```python
from build123d import *

# Parameters (mm, degrees)
F0_W     = 19.05
F0_H     = 184.15
F1_DEPTH = 50.8
F2_W     = 12.7
F2_H     = 25.4
F3_DEPTH = 12.7
F4_W     = 12.7
F4_H     = 25.4
F5_DEPTH = 12.7
F6_R     = 6.34999


# Not quite as in the source:
# - a fillet or chamfer is up to 0.001 mm smaller than in the source, because OpenCascade refuses the exact size


with BuildPart() as f1:
    # F0 (on Top) → F1 (new body)
    with BuildSketch(Plane.XY):
        Rectangle(F0_W, F0_H)
    extrude(amount=-F1_DEPTH)

    # F2 (on face) → F3 (join)
    with BuildSketch(Plane.XZ.offset(92.075)):
        with Locations((0, -25.4)):
            Rectangle(F2_W, F2_H)
    extrude(amount=F3_DEPTH)

    # F4 (on face) → F5 (join)
    with BuildSketch(Plane(origin=(0, 92.075, 0), x_dir=(-1, 0, 0), z_dir=(0, 1, 0))):
        with Locations((0, -25.4)):
            Rectangle(F4_W, F4_H)
    extrude(amount=F5_DEPTH)

    # F6 (radius 6.35 in the source; OpenCascade refuses exactly that, so slightly less here)
    f6_edges = [f1.edges().sort_by_distance(p)[0] for p in [
        (6.35, 98.425, -12.7),
        (-6.35, 98.425, -12.7),
        (-6.35, 98.425, -38.1),
        (6.35, 98.425, -38.1),
        (-6.35, -98.425, -12.7),
        (6.35, -98.425, -12.7),
        (-6.35, -98.425, -38.1),
        (6.35, -98.425, -38.1),
    ]]
    fillet(f6_edges, radius=F6_R)


solid = f1.part
```
Can you work these out from the model? Positions are in its coordinate system, mm. A direction names the side the tool comes from. Round coordinates to 2 decimals unless told otherwise and drop trailing zeros. Loops run counter-clockwise (first coordinate to the right, second up) from the corner with the lowest first, then second, coordinate; pieces in that order, holes last. Notation, with made-up numbers: (25, 7) -> (78, 7) arc R27 ccw to (78, 37) -> close; hole circle Ø2 at (0.25, 44). An arc over 180 degrees is marked (long way). One line per item, written item: value. Start each with the question number.
1. For faces 1 (the cylindrical face through (4.54, 98.51, -36.19)), 2 (the cylindrical face through (-4.44, -98.51, -36.29)), 3 (the flat face through (-6.5, 92.075, -25)), 4 (the cylindrical face through (-4.44, -98.51, -14.51)), 5 (the cylindrical face through (4.44, -98.51, -36.29)), which set-ups out of +Z, -Z, +X, -X, +Y, -Y let a thin tool reach every point of the face, with its end or its side?
2. If we section it at A-A, the plane z = -27.5: Write out the boundary of the cut face in (x, y) (3 decimals).
3. If we section it at B-B, the plane x = 2.25: Write out the boundary of the cut face in (y, z) (3 decimals).
4. For pin 1 (10 mm diameter, centred on y = 98.5, z = -27.5, fed in from -X); pin 2 (6.5 mm diameter, centred on y = -95.5, z = -24, fed in from +X), each with a flat end and sliding along its axis, tell me the tip position at first contact or that it passes through.
5. If I drill on probe 1 along Y at (x, z) = (-7, -3) (3 decimals); probe 2 along Z at (x, y) = (1, 94), over which ranges is the centre line in solid material (lowest first)?
6. If we section it at C-C, the plane z = -42: Write out the boundary of the cut face in (x, y) (3 decimals).
Calculated:
1. face 1: -Z, +X, +Y
1. face 2: -Z, -X, -Y
1. face 3: +Y
1. face 4: +Z, -X, -Y
1. face 5: -Z, +X, -Y
2. outline: (-9.525, -92.075) -> (-6.35, -92.075) -> (-6.35, -104.775) -> (6.35, -104.775) -> (6.35, -92.075) -> (9.525, -92.075) -> (9.525, 92.075) -> (6.35, 92.075) -> (6.35, 104.775) -> (-6.35, 104.775) -> (-6.35, 92.075) -> (-9.525, 92.075) -> close
3. outline: (-104.775, -37.688) -> (-92.075, -37.688) -> (-92.075, -50.8) -> (92.075, -50.8) -> (92.075, -37.688) -> (104.775, -37.688) -> (104.775, -13.112) -> (92.075, -13.112) -> (92.075, 0) -> (-92.075, 0) -> (-92.075, -13.112) -> (-104.775, -13.112) -> close
4. pin 1: stops at x = -6.35
4. pin 2: stops at x = 6.35
5. probe 1: y = -92.075 to 92.075
5. probe 2: z = -38.02 to -12.78
6. outline: (-9.525, -92.075) -> (9.525, -92.075) -> (9.525, 92.075) -> (-9.525, 92.075) -> close
